```python
from build123d import *

# Parameters (mm, degrees)
F1_DEPTH = 1.5
F2_R     = 4
F3_DEPTH = 5.4
F4_R     = 3


with BuildPart() as f1:
    # F0 (on Top) → F1 (new body)
    with BuildSketch(Plane.XY):
        with BuildLine():
            Line((9.95, -4.314368), (9.95, 4.314368))
            ThreePointArc((9.95, 4.314368), (6.538492, 3.775), (8.711352, 6.459769))
            Line((8.711352, 6.459769), (1.238648, 10.774137))
            ThreePointArc((1.238648, 10.774137), (0, 7.55), (-1.238648, 10.774137))
            Line((-1.238648, 10.774137), (-8.711352, 6.459769))
            ThreePointArc((-8.711352, 6.459769), (-6.538492, 3.775), (-9.95, 4.314368))
            Line((-9.95, 4.314368), (-9.95, -4.314368))
            ThreePointArc((-9.95, -4.314368), (-6.538492, -3.775), (-8.711352, -6.459769))
            Line((-8.711352, -6.459769), (-1.238648, -10.774137))
            ThreePointArc((-1.238648, -10.774137), (0, -7.55), (1.238648, -10.774137))
            Line((1.238648, -10.774137), (8.711352, -6.459769))
            ThreePointArc((8.711352, -6.459769), (6.538492, -3.775), (9.95, -4.314368))
        make_face()
    extrude(amount=-F1_DEPTH)

    # F2 (on face) → F3 (join)
    with BuildSketch(Plane.XY):
        Circle(F2_R)
    extrude(amount=F3_DEPTH)

    # F4
    f4_edges = [f1.edges().sort_by_distance(p)[0] for p in [
        (-4, 0, 5.4),
    ]]
    fillet(f4_edges, radius=F4_R)


solid = f1.part
```
Design review of the part built by this model. Coordinates are the model's own, in mm. A direction names the side the tool comes from. Give positions to 0.01 mm unless a question says otherwise; leave off trailing zeros. Write each loop counter-clockwise with the first axis right and the second up, starting at its lowest first coordinate (ties: lowest second). Pieces come first, ordered by that corner, then holes. Notation, with made-up numbers: (42.25, 16) - (80.25, 16) arc R14 cw to (80.25, 35) - close; hole circle Ø5 at (28.25, -18). An arc over 180 degrees is marked (long way). Return JSON: item names as keys, results as strings. Group by question number.
(1) We need section A-A, the plane y = -9.4. Give the boundary of the cut face in (x, z), then the cut area to 3 significant figures.
(2) Machinability: for faces 5 (the flat face through (4.3, 0.2, 0)), 6 (the cylindrical face through (-6.57, -3.72, -0.74)), which of the approach directions +Z, -Z, +X, -X, +Y, -Y give a long, thin tool a straight path to every point of the face, cutting with its end or side? Answer none if there is none.
(3) Mouldability with a two-part tool opening along Y and no side actions: class faces 1 (the flat face through (-4.92, 8.65, -0.74)), 2 (the flat face through (4.92, -8.65, -0.74)), 3 (the flat face through (0, 0, -1.5)), 4 (the cylindrical face through (0.06, 7.55, -0.74)) as +Y half, -Y half, draft (parallel to the pull), parting line (faces both ways), or undercut.
(4) We need section B-B, the plane x = -7.5. Give the boundary of the cut face in (y, z).
(5) We need section D-D, the plane y = -3.75. Give the number of separate pieces and of enclosed holes in the cut face, then the cut area to 3 significant figures.
(6) Insertion check: pin 1 (6 mm diameter, centred on x = 0, y = 9.4, fed in from -Z); pin 2 (5 mm diameter, centred on x = 2.5, y = 7, fed in from +Z); pin 3 (4 mm diameter, centred on y = 7.5, z = 0, fed in from +X); pin 4 (2 mm diameter, centred on x = 8.14, y = 4.7, fed in from +Z). Each pin has a flat end and moves straight along its axis. Give the tip position at first contact, or say it passes through.
(7) We need section C-C, the plane z = -0.5. Give the boundary of the cut face in (x, y), then the cut area to 3 significant figures.
(8) To check wall thickness, follow probe 1 along X at (y, z) = (-4.7, -0.95); probe 2 along Z at (x, y) = (-3.25, 7); probe 3 along X at (y, z) = (9.4, -0.65). State the ranges of each line that lie inside material, in increasing order.
Reported:
{
 "1": {"outline": "(-3.62, -1.5) - (-1.85, -1.5) - (-1.85, 0) - (-3.62, 0) - close; (1.85, -1.5) - (3.62, -1.5) - (3.62, 0) - (1.85, 0) - close", "area": "5.31 mm2"},
 "2": {"face 5": "+Z", "face 6": "+Z, -Z"},
 "3": {"face 1": "+Y half", "face 2": "-Y half", "face 3": "draft", "face 4": "undercut"},
 "4": {"outline": "(-7.16, -1.5) - (-6.44, -1.5) - (-6.44, 0) - (-7.16, 0) - close; (-2.96, -1.5) - (2.96, -1.5) - (2.96, 0) - (-2.96, 0) - close; (6.44, -1.5) - (7.16, -1.5) - (7.16, 0) - (6.44, 0) - close"},
 "5": {"separate pieces": "3", "enclosed holes": "0", "area": "29.6 mm2"},
 "6": {"pin 1": "stops at z = -1.5", "pin 2": "stops at z = 0", "pin 3": "stops at x = 8.71", "pin 4": "passes through"},
 "7": {"outline": "(-9.95, -4.31) arc R1.85 cw (long way) to (-8.71, -6.46) - (-1.24, -10.77) arc R1.85 cw (long way) to (1.24, -10.77) - (8.71, -6.46) arc R1.85 cw (long way) to (9.95, -4.31) - (9.95, 4.31) arc R1.85 cw (long way) to (8.71, 6.46) - (1.24, 10.77) arc R1.85 cw (long way) to (-1.24, 10.77) - (-8.71, 6.46) arc R1.85 cw (long way) to (-9.95, 4.31) - close", "area": "278 mm2"},
 "8": {"probe 1": "x = -6.29 to 6.29", "probe 2": "z = -1.5 to 0", "probe 3": "x = -3.62 to -1.85, 1.85 to 3.62"}
}
